from build123d import *

# Parameters (mm, degrees)
M4_CLEARANCE_HOLE1_D  = 4.5
F_3_0MM_DOWEL_HOLE1_D = 3
SKETCH9_R             = 19
SKETCH9_R_2           = 17.5
CUT_EXTRUDE1_DEPTH    = 29.182441342


with BuildPart() as part:
    # Sketch1 → Revolve1 (revolve)
    with BuildSketch(Plane(origin=(0, 0, 0), x_dir=(1, 0, 0), z_dir=(0, 1, 0))):
        Polygon((19, 8.5), (19, 7.5), (17.5, 7.5), (17.5, 1), (19, 1), (19, 0), (10.5, 0), (10.5, -4), (0, -4), (0, 8.5), align=None)
    revolve(axis=Axis((0, 0, 4), (0, 0, -1)))

    # M4 Clearance Hole1 (through all)
    with Locations(Plane(origin=(0, 0, -8.5), x_dir=(-1, 0, 0), z_dir=(0, 0, -1))):
        with Locations((-12.124355653, 7), (0, 14), (12.124355653, 7), (12.124355653, -7), (0, -14), (-12.124355653, -7)):
            Hole(M4_CLEARANCE_HOLE1_D / 2)

    # Ø3.0mm Dowel Hole1 (through all)
    with Locations(Plane(origin=(0, 0, -8.5), x_dir=(-1, 0, 0), z_dir=(0, 0, -1))):
        with Locations((14, 0), (-14, 0)):
            Hole(F_3_0MM_DOWEL_HOLE1_D / 2)

    # Sketch9 → Cut-Extrude1 (cut, through all)
    with BuildSketch(Plane.XY):
        Circle(SKETCH9_R)
        Circle(SKETCH9_R_2, mode=Mode.SUBTRACT)
    extrude(amount=-CUT_EXTRUDE1_DEPTH, mode=Mode.SUBTRACT)


solid = part.part
Input: part model. Units: mm. Frame: model coordinates. A direction names the side the tool comes from. Coordinates: 2 decimals unless noted, no trailing zeros. Order: outer loops, then holes, each group sorted by start corner. A loop starts at its lowest first (then second) coordinate and runs counter-clockwise, first axis right, second up. Notation, with made-up numbers: M -36.5,54.5 L -6.5,54.5 A29 cw -6.5,89.5 Z; hole C 59,1.5 d3. An arc over 180 degrees is marked long. Answer in a Markdown table with one row per item.
(1) Access query for faces 5 (the cylindrical face through (-10.915, 8.897, -4.19)), 6 (the flat face through (8, 8, 0)). Directions: +Z, -Z, +X, -X, +Y, -Y. A direction counts if a zero-diameter tool reaches every point of the face in a straight line with its end or side. Return the directions, or none.
Numbers:
| item | result |
|---|---|
| face 5 | +Z, -Z |
| face 6 | +Z |
(2) Material intervals for line 1 (Y direction, x = 0, z = -6.25); line 2 (Y direction, x = 12, z = -1.5); line 3 (X direction, y = 5, z = -1), sorted ascending. Write a range as [from, to].
Numbers:
| item | result |
|---|---|
| line 1 | y = [-17.5, -16.25], [-11.75, 11.75], [16.25, 17.5] |
| line 2 | y = [-12.74, -9.25], [-4.75, 4.75], [9.25, 12.74] |
| line 3 | x = [-16.77, -13.16], [-11.09, 11.09], [13.16, 16.77] |
(3) Section query A-A, the plane y = 0. Output: boundary loops of the cut face in (x, z).
Numbers:
| item | result |
|---|---|
| outline | M -17.5,-8.5 L -15.5,-8.5 L -15.5,0 L -17.5,0 Z; M -12.5,-8.5 L 12.5,-8.5 L 12.5,0 L 10.5,0 L 10.5,4 L -10.5,4 L -10.5,0 L -12.5,0 Z; M 15.5,-8.5 L 17.5,-8.5 L 17.5,0 L 15.5,0 Z |
(4) Section query B-B, the plane y = -14. Output: boundary loops of the cut face in (x, z).
Numbers:
| item | result |
|---|---|
| outline | M -10.5,-8.5 L -2.25,-8.5 L -2.25,0 L -10.5,0 Z; M 2.25,-8.5 L 10.5,-8.5 L 10.5,0 L 2.25,0 Z |
(5) Section query C-C, the plane x = -15. Output: boundary loops of the cut face in (y, z), plus the area to 3 significant figures.
Numbers:
| item | result |
|---|---|
| outline | M -9.01,-8.5 L -1.12,-8.5 L -1.12,0 L -9.01,0 Z; M 1.12,-8.5 L 9.01,-8.5 L 9.01,0 L 1.12,0 Z |
| area | 134 mm^2 |
(6) Contact query for flat-ended pins moving along their axis: pin 1 Ø3 at (x, z) = (-5.5, 1) entering from +Y; pin 2 Ø7 at (x, y) = (0, -14) entering from -Z; pin 3 Ø4 at (x, z) = (5.5, -6.5) entering from +Y; pin 4 Ø6 at (x, y) = (-12.12, 7) entering from +Z. Output: stop coordinate, or through.
Numbers:
| item | result |
|---|---|
| pin 1 | stops at y = 16.94 |
| pin 2 | stops at z = -8.5 |
| pin 3 | stops at y = 17.15 |
| pin 4 | stops at z = 0 |
(7) Section query D-D, the plane z = -4.5. Give the number of separate pieces and of enclosed holes in the cut face, plus the area to 3 significant figures.
Numbers:
| item | result |
|---|---|
| separate pieces | 1 |
| enclosed holes | 8 |
| area | 853 mm^2 |
(8) Draft query along X for faces 1 (the cylindrical face through (-0.488, -16.196, -4.19)), 2 (the flat face through (0, 0, 4)), 3 (the cylindrical face through (-13.887, -10.648, -4.19)), 4 (the cylindrical face through (14.27, 7.68, -4.19)). Return one class per face: pulls with the +X half, pulls with the -X half, needs draft (parallel to the pull), parting line crosses it, or undercut.
Numbers:
| item | result |
|---|---|
| face 1 | undercut |
| face 2 | needs draft |
| face 3 | parting line crosses it |
| face 4 | undercut |
